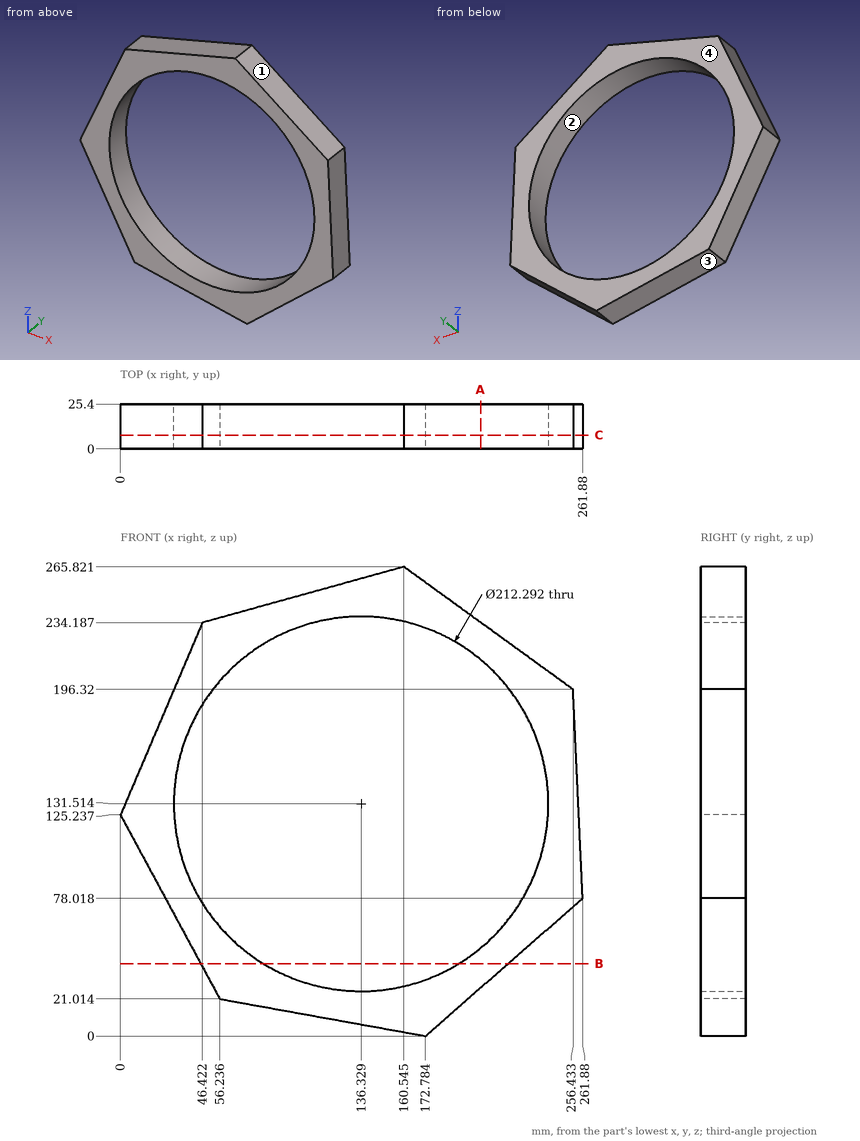
Verification items for this drawing (mm, ordinates from the low corner). Give positions to 0.01 mm unless a question says otherwise; leave off trailing zeros. Write each loop counter-clockwise with the first axis right and the second up, starting at its lowest first coordinate (ties: lowest second). Pieces come first, ordered by that corner, then holes. Notation, with made-up numbers: (30.25, 63.5) - (89.25, 63.5) arc R24 cw to (89.25, 74.5) - close; hole circle Ø10 at (-21, 46.25). An arc over 180 degrees is marked (long way). Answer as a JSON object with one key per item and string values. Group by question number.
1) Sectioned sample at A-A (x = 204). Record the cut outline in (y, z) (1 decimal).
2) Depth check by flat-ended pin: P1, Ø8, axis at y = 16, z = 91, coming from the -X side (1 decimal); P2, Ø2, axis at x = 176, y = 4, coming from the +Z side (1 decimal); P3, Ø2, axis at y = 14, z = 175.5, coming from the -X side; P4, Ø2, axis at x = 126, z = 27.5, coming from the +Y side. Enter the tip coordinate at first touch or a pass-through.
3) Sectioned sample at B-B (z = 41). Record the cut outline in (x, y) (1 decimal), then the cut area to 3 significant figures.
4) Thickness scan on probe 1 along Z at (x, y) = (141, 5.75); probe 2 along Z at (x, y) = (185.5, 4) (1 decimal); probe 3 along X at (y, z) = (16, 222) (1 decimal). Record the ranges inside material, lowest first. Write a range as from..to.
5) Sectioned sample at C-C (y = 7.75). Record the cut outline in (x, z) (1 decimal).
6) Release check for a two-part mould opening along Z. For the marked faces 1, 2, 3 and 4 record: pulls with the +Z half, pulls with the -Z half, needs draft (parallel to the pull), parting line crosses it, or undercut.
Geometry results:
{
 "1": {"outline": "(0, 27.3) - (25.4, 27.3) - (25.4, 49.7) - (0, 49.7) - close; (0, 213.3) - (25.4, 213.3) - (25.4, 234.3) - (0, 234.3) - close"},
 "2": {"P1": "stops at x = 16.3", "P2": "stops at z = 255.3", "P3": "stops at x = 20.99", "P4": "passes through"},
 "3": {"outline": "(45.5, 0) - (80.9, 0) - (80.9, 25.4) - (45.5, 25.4) - close; (191.8, 0) - (219.6, 0) - (219.6, 25.4) - (191.8, 25.4) - close", "area": "1,610 mm^2"},
 "4": {"probe 1": "z = 5.73..25.47, 237.56..260.4", "probe 2": "z = 11.1..37.4, 225.6..247.7", "probe 3": "x = 41.2..80.8, 191.8..221"},
 "5": {"outline": "(0, 125.2) - (56.2, 21) - (172.8, 0) - (261.9, 78) - (256.4, 196.3) - (160.5, 265.8) - (46.4, 234.2) - close; hole circle Ø212.3 at (136.3, 131.5)"},
 "6": {"face 1": "pulls with the +Z half", "face 2": "undercut", "face 3": "pulls with the -Z half", "face 4": "needs draft"}
}
